```python
from build123d import *

# Parameters (mm, degrees)
F0_W     = 12.7
F0_H     = 3.175
F0_W_2   = 3.175
F0_H_2   = 12.7
F1_DEPTH = 3.175


with BuildPart() as f1:
    # F0 (on Top) → F1 (new body)
    with BuildSketch(Plane.XY):
        Polygon((-12.7, 22.225), (-22.225, 22.225), (-22.225, 12.7), (-22.225, 0), (-22.225, -12.7), (-22.225, -22.225), (-12.7, -22.225), (0, -22.225), (12.7, -22.225), (22.225, -22.225), (22.225, -12.7), (22.225, 0), (22.225, 12.7), (22.225, 22.225), (12.7, 22.225), (0, 22.225), align=None)
        with Locations((-6.35, 23.8125)):
            Rectangle(F0_W, F0_H)
        with Locations((6.35, 23.8125)):
            Rectangle(F0_W, F0_H)
        with Locations((23.8125, 6.35)):
            Rectangle(F0_W_2, F0_H_2)
        with Locations((23.8125, -6.35)):
            Rectangle(F0_W_2, F0_H_2)
        with Locations((6.35, -23.8125)):
            Rectangle(F0_W, F0_H)
        with Locations((-6.35, -23.8125)):
            Rectangle(F0_W, F0_H)
        with Locations((-23.8125, -6.35)):
            Rectangle(F0_W_2, F0_H_2)
        with Locations((-23.8125, 6.35)):
            Rectangle(F0_W_2, F0_H_2)
    extrude(amount=F1_DEPTH)


solid = f1.part
```
Input: part model. Units: mm. Frame: model coordinates. A direction names the side the tool comes from. Give positions to 0.01 mm unless a question says otherwise; leave off trailing zeros. Order: outer loops, then holes, each group sorted by start corner. A loop starts at its lowest first (then second) coordinate and runs counter-clockwise, first axis right, second up. Notation, with made-up numbers: M 88.25,54.5 L 124.25,54.5 A28 ccw 124.25,73.5 Z; hole C -27,82.5 d8. An arc over 180 degrees is marked long. Return JSON: item names as keys, results as strings.
Item 1: Cut plane B-B (x = 14.5). Return loops of the section in (y, z) (3 decimals).
Solutions:
{"outline": "M -22.225,0 L 22.225,0 L 22.225,3.175 L -22.225,3.175 Z"}
Item 2: Cut plane A-A (z = 2.3). Return loops of the section in (x, y) (3 decimals).
Solutions:
{"outline": "M -25.4,-12.7 L -22.225,-12.7 L -22.225,-22.225 L -12.7,-22.225 L -12.7,-25.4 L 12.7,-25.4 L 12.7,-22.225 L 22.225,-22.225 L 22.225,-12.7 L 25.4,-12.7 L 25.4,12.7 L 22.225,12.7 L 22.225,22.225 L 12.7,22.225 L 12.7,25.4 L -12.7,25.4 L -12.7,22.225 L -22.225,22.225 L -22.225,12.7 L -25.4,12.7 Z"}
Item 3: First-contact query: P1, Ø5, axis at x = 3, y = 18.5, coming from the -Z side; P2, Ø1, axis at x = -23.5, z = 2.5, coming from the +Y side; P3, Ø1.6, axis at y = 24.5, z = 1.5, coming from the -X side; P4, Ø1, axis at y = 18, z = 2, coming from the -X side (3 decimals). Flat tips, straight axial feed; report the tip coordinate or a pass-through.
Solutions:
{"P1": "z = 0", "P2": "y = 12.7", "P3": "x = -12.7", "P4": "x = -22.225"}
Item 4: Access query for faces 1 (the flat face through (22.225, -18, 2)), 2 (the flat face through (24, 12.7, 2)), 3 (the flat face through (-24, 12.7, 2)). Directions: +Z, -Z, +X, -X, +Y, -Y. A direction counts if a zero-diameter tool reaches every point of the face in a straight line with its end or side. Return the directions, or none.
Solutions:
{"face 1": "+Z, -Z, +X, -Y", "face 2": "+Z, -Z, +X, +Y", "face 3": "+Z, -Z, -X, +Y"}
Item 5: Ray query, probe 1 along Y at (x, z) = (-15, 0.75) (3 decimals); probe 2 along X at (y, z) = (-23, 0.55). Return the intervals inside material, ascending.
Solutions:
{"probe 1": "-22.225 to 22.225", "probe 2": "-12.7 to 12.7"}
